Autodesk Inventor part; units mm, degrees
ref_plane "Work Plane1" through (236.99, 0, 0) normal (1, 0, 0) x (0, 0, -1)
ref_plane "Work Plane2" through (236.99, 52.5583, -19.3295) normal (0, 0.9385405, -0.3451692) x (-1, 0, 0)
ref_plane "Work Plane3" through (128.29, 0, 0) normal (-1, 0, 0) x (0, 0, 1)
sketch "Sketch1" plane through (0, 0, 0) normal (0, 1, 0) x (-1, 0, 0)
  line L0 (0, 0) -> (-303.89, 0)
  line L1 (0, 0) -> (0, -12.7)
  line L2 (0, -12.7) -> (-87.53, -12.7)
  line L3 (-87.53, -12.7) -> (-87.53, -17.315)
  line L4 (-87.53, -17.315) -> (-50.03, -17.315)
  line L5 (-50.03, -17.315) -> (-50.03, -20.525)
  line L6 (-50.03, -20.525) -> (-47.53, -20.525)
  line L7 (-47.53, -20.525) -> (-47.53, -27.45)
  line L8 (-47.53, -27.45) -> (-50.63, -27.45)
  line L9 (-50.63, -27.45) -> (-52.53, -19.05)
  line L10 (-52.53, -19.05) -> (-81.13, -19.05)
  line L11 (-81.13, -19.05) -> (-81.13, -37.8)
  line L12 (-81.13, -37.8) -> (-119.39, -37.8)
  line L13 (-119.39, -37.8) -> (-119.39, -25.5)
  line L14 (-119.39, -25.5) -> (-134.29, -37.635)
  line L15 (-134.29, -37.635) -> (-134.29, -43.07)
  line L16 (-134.29, -43.07) -> (-137.79, -43.07)
  line L17 (-137.79, -43.07) -> (-137.79, -43.28)
  line L18 (-137.79, -43.28) -> (-139.89, -43.28)
  line L19 (-139.89, -43.28) -> (-139.89, -43.175)
  line L20 (-139.89, -43.175) -> (-236.29, -43.175)
  line L21 (-236.29, -43.175) -> (-236.29, -56)
  line L22 (-236.29, -56) -> (-238.99, -56)
  line L23 (-238.99, -56) -> (-238.99, 0)
  line L24 (-251.3, 0) -> (-251.3, -38.15)
  line L25 (-251.3, -38.15) -> (-291.54, -38.15)
  line L26 (-291.54, -38.15) -> (-291.54, -7.165)
  line L27 (-291.54, -7.165) -> (-303.89, -7.165)
  line L28 (-303.89, -7.165) -> (-303.89, 0)
  line L29 (-238.99, -38) -> (-251.3, -38)
  line L30 (-251.3, -38) -> (-251.3, 0)
  line L31 (-251.3, 0) -> (-238.99, 0)
  line L32 (-238.99, 0) -> (-238.99, -38)
  dimension "d0" = 303.89
  dimension "d1" = 12.7
  dimension "d2" = 87.53
  dimension "d3" = 4.615
  dimension "d4" = 37.5
  dimension "d5" = 3.21
  dimension "d6" = 2.5
  dimension "d7" = 27.45
  dimension "d8" = 3.1
  dimension "d9" = 5
  dimension "d10" = 19.05
  dimension "d11" = 30.5
  dimension "d12" = 37.8
  dimension "d13" = 38.26
  dimension "d14" = 12.3
  dimension "d16" = 14.9
  dimension "d17" = 37.635
  dimension "d18" = 43.07
  dimension "d19" = 3.5
  dimension "d20" = 43.28
  dimension "d21" = 2.1
  dimension "d22" = 43.175
  dimension "d24" = 56
  dimension "d25" = 104.7
  dimension "d26" = 12.31
  dimension "d27" = 157.25
  dimension "d28" = 38.15
  dimension "d29" = 90
  dimension "d30" = 7.165
  dimension "d31" = 12.35
  dimension "d54" = 2.7
  dimension "d55" = 38
  dimension "d77" = 25.5
  dimension "d78" = 102
revolve "Revolution1" add sketch "Sketch1" angle 360 about axis through (0, 0, 0) along (1, 0, 0)
ref_plane "Work Plane1" through (236.99, 0, 0) normal (1, 0, 0) x (0, 0, -1)
ref_plane "Work Plane2" through (236.99, 52.5583, -19.3295) normal (0, 0.9385405, -0.3451692) x (-1, 0, 0)
sketch "Sketch6" plane through (238.99, 0, 0) normal (1, 0, 0) x (0, 0, -1)
  line L0 (44.25, -25.5477) -> (-44.25, -25.5477)
  line L1 (-44.25, -25.5477) -> (0, 51.0955)
  line L2 (0, 51.0955) -> (44.25, -25.5477)
  circle A0 centre (0, 51.0955) radius 2
  circle A1 centre (44.25, -25.5477) radius 2
  circle A2 centre (-44.25, -25.5477) radius 2
  point P0 (0, 0)
  point P1 (0, 0)
  dimension "d56" = 4
  dimension "d57" = 88.5
extrude "Extrusion3" cut sketch "Sketch6" against normal up to surface (2.7 mm away) contours A2 L1 L0 | L0 L1 A2 | A1 L2 L0 | L0 L2 A1 | A0 L2 L1 | L1 L2 A0
ref_plane "Work Plane3" through (128.29, 0, 0) normal (-1, 0, 0) x (0, 0, 1)
sketch "Sketch7" plane through (128.29, 0, 0) normal (-1, 0, 0) x (0, 0, 1)
  circle A0 centre (0, 51.0955) radius 2
  circle A1 centre (0, 0) radius 25.5
  circle A2 centre (0, 0) radius 37.635
  circle A3 centre (0, 0) radius 32.635 construction
  circle A4 centre (0, 32.635) radius 2
  circle A5 centre (25.2927, 20.6234) radius 2
  dimension "d61" = 5
  dimension "d62" = 4
  dimension "d64" = 28
extrude "Extrusion4" add sketch "Sketch7" along normal mid plane 3 contours A4 | A5
ref_plane "Work Plane4" through (226.29, 0, 0) normal (-1, 0, 0) x (0, 0, 1)
sketch "Sketch8" plane through (226.29, 0, 0) normal (-1, 0, 0) x (0, 0, 1)
  circle A0 centre (0, 0) radius 43.175
  circle A1 centre (0, 0) radius 43.175
  circle A2 centre (-44.25, -25.5477) radius 2
  line L0 (-44.25, -25.5477) -> (-37.3906, -21.5875) construction
  point P0 (-23.6509, -36.1209)
  dimension "d68" = 20
ref_plane "Work Plane5" through (226.29, -36.1209, -23.6509) normal (0, -0.8366152, -0.547791) x (1, 0, 0)
sketch "Sketch9" plane through (226.29, -36.1209, -23.6509) normal (0, -0.8366152, -0.547791) x (1, 0, 0)
  circle A0 centre (0, 0) radius 3.1
  point P0 (-226.29, 0)
  dimension "d69" = 6.2
extrude "Extrusion5" add sketch "Sketch9" along normal blind 26 and the other way blind 1
sketch "Sketch10" plane through (226.29, -57.8729, -37.8934) normal (0, -0.8366152, -0.547791) x (1, 0, 0)
  circle A0 centre (0, 0) radius 3.1
  circle A1 centre (0, 0) radius 7
  point P0 (-226.29, 0)
  dimension "d74" = 14
extrude "Extrusion6" add sketch "Sketch10" against normal blind 13 contours A0 | A1
properties part number "STI Hybrid 98 Cryocooler - Full Flange"
Read the model definition and answer for the solid it produces. Units are mm, in the model's axes. A direction names the side the tool comes from. Coordinates: 2 decimals unless noted, no trailing zeros. Write each loop counter-clockwise with the first axis right and the second up, starting at its lowest first coordinate (ties: lowest second). Pieces come first, ordered by that corner, then holes. Notation, with made-up numbers: (-3.5, 79.5) -> (10.5, 79.5) arc R29 cw to (10.5, 115.5) -> close; hole circle Ø11 at (-16.5, 33.25). An arc over 180 degrees is marked (long way). Answer as a JSON object with one key per item and string values.
Q1. Consider line 1 (Y direction, x = 65.5, z = 0) (3 decimals); line 2 (Y direction, x = 48.25, z = 0) (3 decimals); line 3 (X direction, y = 15, z = -4.5). Determine where each line is inside the solid, lowest interval first. Write a range as [from, to].
The answers:
{"line 1": "y = [-19.05, -17.315], [-12.7, 12.7], [17.315, 19.05]", "line 2": "y = [-27.45, -20.525], [-12.7, 12.7], [20.525, 27.45]", "line 3": "x = [87.53, 291.54]"}
Q2. Determine the mould class of faces 4 (the cylindrical face through (237.66, -21.45, -51.73)), 5 (the flat face through (303.89, 0, 0)), 6 (the flat face through (50.03, -14, 11)) for opening direction Z: pulls with the +Z half, pulls with the -Z half, needs draft (parallel to the pull), parting line crosses it, or undercut.
The answers:
{"face 4": "parting line crosses it", "face 5": "needs draft", "face 6": "undercut"}
Q3. A tool of negligible diameter and unlimited length cuts with its end or side. For faces 1 (the flat face through (81.13, 9, 17)), 2 (the cylindrical face through (297.801, 0.315, 7.158)), 3 (the flat face through (47.53, -18.2, -10)), from which of +Z, -Z, +X, -X, +Y, -Y can it reach the whole face along a straight path? Write none if from no direction.
The answers:
{"face 1": "none", "face 2": "+X", "face 3": "-X"}
Q4. Flat-ended cylindrical pins translate along their axes: pin 1 Ø3 at (x, y) = (202, -45) entering from +Z; pin 2 Ø3 at (x, z) = (259.5, 14.5) entering from +Y; pin 3 Ø2 at (y, z) = (21, 26.5) entering from +X; pin 4 Ø8 at (x, y) = (214.5, -42.5) entering from -Z. Find the tip coordinate at first contact, or state that the pin passes through.
The answers:
{"pin 1": "passes through", "pin 2": "stops at y = 35.87", "pin 3": "stops at x = 291.54", "pin 4": "stops at z = -19.54"}
Q5. The part is cut by section B-B on x = 158.5. Give the vertices of the cut face in (y, z) (3 decimals).
The answers:
{"outline": "circle Ø86.35 at (0, 0)"}
Q6. The part is cut by section A-A on x = 265.5. Give the vertices of the cut face in (y, z), then the cut area to 3 significant figures.
The answers:
{"outline": "circle Ø76.3 at (0, 0)", "area": "4,570 mm2"}
